Autodesk Inventor part; units mm, degrees
ref_plane "YZ Plane" through (0, 0, 0) normal (1, 0, 0) x (0, 1, 0)
ref_plane "XZ Plane" through (0, 0, 0) normal (0, 1, 0) x (-1, 0, 0)
ref_plane "XY Plane" through (0, 0, 0) normal (0, 0, 1) x (1, 0, 0)
sketch "Esquisse1" plane through (0, 0, 0) normal (0, 1, 0) x (-1, 0, 0)
  circle A0 centre (0, 0) radius 15.5
  dimension "d0" = 31
extrude "Extrusion1" add sketch "Esquisse1" along normal blind 7
fillet "Congé1" radius 2 1 edges at (15.5, 7, 0)
fillet "Congé2" radius 2 1 edges at (15.5, 0, 0)
sketch "Esquisse3" plane through (0, 7, 0) normal (0, 1, 0) x (1, 0, 0)
  circle A0 centre (0, 0) radius 12.5
  dimension "d10" = 25
extrude "Extrusion2" cut sketch "Esquisse3" against normal blind 10
thread "Filetage3"
properties part number "Anneau interm"
Verification items for the finished model (mm, model axes). Coordinates: 2 decimals unless noted, no trailing zeros. Loops run counter-clockwise (first coordinate to the right, second up) from the corner with the lowest first, then second, coordinate; pieces in that order, holes last. Notation, with made-up numbers: (15.25, 86) - (64.25, 86) arc R25 ccw to (64.25, 112) - close; hole circle Ø10 at (-33.5, 8.25). An arc over 180 degrees is marked (long way). Return JSON: item names as keys, results as strings.
1. Mould release check, pull along Z, two halves, no side actions. Record for faces 1 (the cylindrical face through (11.923, 3.549, -3.755)), 2 (the cylindrical face through (2.018, 3.479, -15.368)), 3 (the flat face through (-9, 0, -9)): +Z half, -Z half, draft (parallel to the pull), parting line (faces both ways), or undercut.
Established:
{"face 1": "undercut", "face 2": "parting line", "face 3": "draft"}
2. Section check A-A, the plane z = 0. Record the boundary of the cut face in (x, y), then the cut area to 3 significant figures.
Established:
{"outline": "(-15.5, 2) arc R2 ccw to (-13.5, 0) - (-12.5, 0) - (-12.5, 7) - (-13.5, 7) arc R2 ccw to (-15.5, 5) - close; (12.5, 0) - (13.5, 0) arc R2 ccw to (15.5, 2) - (15.5, 5) arc R2 ccw to (13.5, 7) - (12.5, 7) - close", "area": "38.6 mm2"}
3. Thickness scan on L1, parallel to Z at x = 0, y = 3.5; L2, parallel to Y at x = 13.5, z = -1.5; L3, parallel to Z at x = -5.5, y = 5. Record the ranges inside material, lowest first.
Established:
{"L1": "z = -15.5 to -12.5, 12.5 to 15.5", "L2": "y = 0 to 7", "L3": "z = -14.49 to -11.22, 11.22 to 14.49"}
4. Section check D-D, the plane y = 5.75. Record the boundary of the cut face in (x, z).
Established:
{"outline": "circle Ø30.71 at (0, 0); hole circle Ø25 at (0, 0)"}
5. Go/stop test with flat-tipped pins: pin 1 (3 mm diameter, centred on y = 6, z = 5, fed in from +X); pin 2 (1.5 mm diameter, centred on y = 1, z = 3.5, fed in from -X); pin 3 (1.5 mm diameter, centred on x = -6, y = 4.5, fed in from -Z). Record where each tip stops, or that it passes through.
Established:
{"pin 1": "stops at x = 15.04", "pin 2": "stops at x = -15.16", "pin 3": "stops at z = -14.58"}
6. Section check B-B, the plane x = 0. Record the boundary of the cut face in (y, z), then the cut area to 3 significant figures.
Established:
{"outline": "(0, -13.5) arc R2 ccw to (2, -15.5) - (5, -15.5) arc R2 ccw to (7, -13.5) - (7, -12.5) - (0, -12.5) - close; (0, 12.5) - (7, 12.5) - (7, 13.5) arc R2 ccw to (5, 15.5) - (2, 15.5) arc R2 ccw to (0, 13.5) - close", "area": "38.6 mm2"}
7. Section check C-C, the plane y = 2.5. Record the boundary of the cut face in (x, z), then the cut area to 3 significant figures.
Established:
{"outline": "circle Ø31 at (0, 0); hole circle Ø25 at (0, 0)", "area": "264 mm2"}
